Part model, mm, in its own coordinate system. A direction names the side the tool comes from. Give positions to 0.01 mm unless a question says otherwise; leave off trailing zeros. Order: outer loops, then holes, each group sorted by start corner. A loop starts at its lowest first (then second) coordinate and runs counter-clockwise, first axis right, second up. Notation, with made-up numbers: M -8,74.25 L 39,74.25 A13 cw 39,92.25 Z; hole C 36.5,-36.5 d5. An arc over 180 degrees is marked long. Answer as a JSON object with one key per item and string values.
from build123d import *

# Parameters (mm, degrees)
F1_DEPTH = 6
F3_D     = 1.8


with BuildPart() as f1:
    # F0 (on Right) → F1 (new body)
    with BuildSketch(Plane.YZ):
        Polygon((-3, 0), (0, 0), (6, 0), (6, 2.5), (0, 2.5), (0, 13.7304612652), (0, 18), (-3, 18), (-3, 12.3315382908), (-8, 10), (-3, 10), align=None)
    extrude(amount=-F1_DEPTH)

    # F3 (through all)
    with Locations(Plane(origin=(0, 0, 0), x_dir=(1, 0, 0), z_dir=(0, 0, -1))):
        with Locations((-3, -4.5)):
            Hole(F3_D / 2)

    # F7: sweep along a path in F6
    with BuildLine(Plane.YZ) as f7_path:
        Line((-3, 14.3315382908), (0, 16.8315382908))
    # F5 (on face) → F7 (sweep, cut)
    with BuildSketch(Plane.XZ.offset(3)):
        with BuildLine():
            ThreePointArc((-3, 12.3315382908), (-1.5857864376, 12.9173247284), (-1, 14.3315382908))
            ThreePointArc((-1, 14.3315382908), (-4.4142135624, 15.7457518531), (-3, 12.3315382908))
        make_face()
    sweep(path=f7_path.line, mode=Mode.SUBTRACT)


solid = f1.part
1. Probe line 1 along X through (y, z) = (4.5, 1.1); line 2 along Y through (x, z) = (-3, 0.65); line 3 along Y through (x, z) = (-5.5, 3). List the from-to ranges inside material, lowest first.
Worked answers:
{"line 1": "x = -6 to -3.9, -2.1 to 0", "line 2": "y = -3 to 3.6, 5.4 to 6", "line 3": "y = -3 to 0"}
2. Cut at D-D on z = 10.5. Give the cut face in (x, y).
Worked answers:
{"outline": "M -6,-6.93 L 0,-6.93 L 0,0 L -6,0 Z"}
3. Which spindle directions (+Z, -Z, +X, -X, +Y, -Y) get a long thin tool onto all of the face, cutting with end or side? Do faces 5 (the flat face through (0, -1, 6)), 6 (the flat face through (-3, 0, 8)), 7 (the flat face through (-3, -6, 10)). Say none if no direction does.
Worked answers:
{"face 5": "+Z, -Z, +X, +Y, -Y", "face 6": "+Z, +X, -X, +Y", "face 7": "-Z, +X, -X, -Y"}
4. Two-plate mould, pull along Y, no slides. Class faces 1 (the cylindrical face through (-3.415, 5.298, 1.267)), 2 (the flat face through (-3, 6, 1)), 3 (the flat face through (-3, 3, 2.5)), 4 (the flat face through (-2.3, -3, 16.5)): +Y half, -Y half, draft (parallel to the pull), parting line (faces both ways), or undercut.
Worked answers:
{"face 1": "undercut", "face 2": "+Y half", "face 3": "draft", "face 4": "-Y half"}
5. Pin check, flat tips, straight feed: P1, Ø4, axis at y = -6.5, z = 5.5, coming from the -X side; P2, Ø2, axis at x = -3.5, z = 6, coming from the -Y side; P3, Ø2, axis at x = -3.5, z = 10, coming from the +Y side; P4, Ø3, axis at x = -3.5, y = -5, coming from the -Z side. Stop position of each tip, or through.
Worked answers:
{"P1": "passes through", "P2": "stops at y = -3", "P3": "stops at y = 0", "P4": "stops at z = 10"}
6. Cut at A-A on y = 4.5. Give the cut face in (x, z), plus the area to 3 significant figures.
Worked answers:
{"outline": "M -6,0 L -3.9,0 L -3.9,2.5 L -6,2.5 Z; M -2.1,0 L 0,0 L 0,2.5 L -2.1,2.5 Z", "area": "10.5 mm^2"}
7. Cut at B-B on x = -0.25. Give the cut face in (y, z), plus the area to 3 significant figures.
Worked answers:
{"outline": "M -8,10 L -3,10 L -3,0 L 6,0 L 6,2.5 L 0,2.5 L 0,18 L -3,18 L -3,12.33 Z", "area": "74.8 mm^2"}
8. Cut at C-C on y = 3. Give the cut face in (x, z).
Worked answers:
{"outline": "M -6,0 L 0,0 L 0,2.5 L -6,2.5 Z"}
